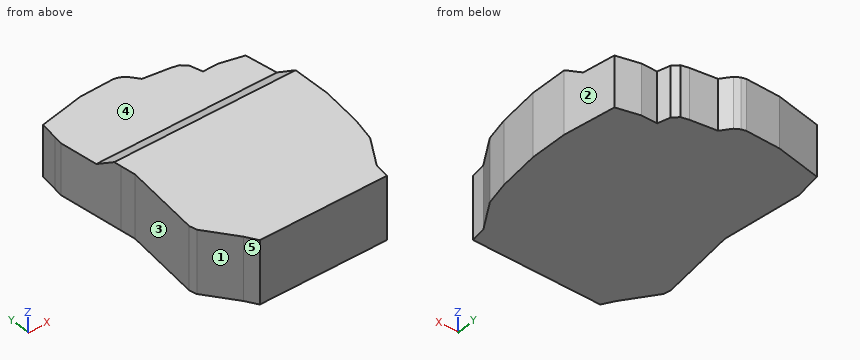
from build123d import *

# Parameters (mm, degrees)
BOSS_EXTRUDE1_DEPTH     = 30
CUT_EXTRUDE2_DEPTH      = 161.362841695
CUT_EXTRUDE2_DEPTH_BACK = 161.362841695


with BuildPart() as part:
    # Sketch1 → Boss-Extrude1 (new body)
    with BuildSketch(Plane.XY):
        Polygon((546.580924534, 9.896085679), (608.250924534, 9.896085679), (609.468725462, 17.325239217), (618.364062826, 31.698748766), (621.209508482, 43.308723045), (623.868380606, 63.224196603), (623.868380606, 81.054488799), (620.357339754, 106.059490311), (609.468725462, 108.728140515), (601.88762533, 108.728140515), (600.342350418, 114.668879106), (597.693307712, 117.244337292), (594.121848564, 118.119653006), (581.623216062, 119.788318601), (578.065152196, 124.442825109), (575.59297034, 125.972784898), (573.39799577, 126.510743097), (557.030037078, 126.118131563), (535.309704018, 121.76025213), (533.883150006, 113.057607434), (533.173455584, 108.728140515), (536.320171406, 77.786869686), (537.054893461, 70.562437811), (532.098682684, 33.439447285), (532.810591456, 29.891185826), (543.388975695, 15.373727724), align=None)
    extrude(amount=BOSS_EXTRUDE1_DEPTH)

    # Sketch2 → Cut-Extrude2 (cut, two sides: drawn at the far end of the back side and taken through both)
    with BuildSketch(Plane(origin=(530, 0, 0), x_dir=(0, 0, -1), z_dir=(1, 0, 0)).offset(-CUT_EXTRUDE2_DEPTH_BACK)):
        Polygon((-24.212, 126.510743097), (-24.212, 90.610743097), (-30, 81.373139386), (-30, 126.510743097), align=None)
    extrude(amount=CUT_EXTRUDE2_DEPTH + CUT_EXTRUDE2_DEPTH_BACK, mode=Mode.SUBTRACT)


solid = part.part
Design review of the part built by this model. Coordinates are the model's own, in mm. Face numbers are marked on the shaded views. A direction names the side the tool comes from. Coordinates: 2 decimals unless noted, no trailing zeros. Loops run counter-clockwise (first coordinate to the right, second up) from the corner with the lowest first, then second, coordinate; pieces in that order, holes last. Notation, with made-up numbers: (11.5, -24) -> (70.5, -24) arc R23 ccw to (70.5, -9) -> close; hole circle Ø9 at (9.5, 83). An arc over 180 degrees is marked (long way). Use a Markdown table: item, result. Add a question column.
Item 1: We need section A-A, the plane z = 9.75. Write out the cut boundary in (x, y).
Item 2: We need section C-C, the plane y = 85. Write out the cut boundary in (x, z).
Item 3: We need section B-B, the plane x = 606.5. Write out the cut boundary in (y, z).
Item 4: Machinability: for the marked faces 4 and 5, which of the approach directions +Z, -Z, +X, -X, +Y, -Y give a long, thin tool a straight path to every point of the face, cutting with its end or side? Answer none if there is none.
Item 5: We need section D-D, the plane x = 561.5. Write out the cut boundary in (y, z).
Item 6: Clearance check with flat-ended pins moving along their axes: P1, Ø5, axis at y = 30.5, z = 8, coming from the -X side; P2, Ø11, axis at x = 586, y = 107.5, coming from the +Z side; P3, Ø8.5, axis at x = 604.5, z = 8, coming from the +Y side. State where each tip first meets the part, or that it passes through.
Item 7: Wall thickness on L1, parallel to Y at x = 607, z = 9.75; L2, parallel to Z at x = 614.5, y = 101; L3, parallel to Y at x = 617, z = 26.75: over which ranges is each line inside the solid? List them lowest first. Write a range as from..to.
Item 8: The part is to be moulded in two halves that separate along Y. For the marked faces 1, 2 and 3, say which applies: +Y half, -Y half, draft (parallel to the pull), parting line (faces both ways), or undercut.
Numbers:
| question | item | result |
|---|---|---|
| 1 | outline | (532.1, 33.44) -> (532.81, 29.89) -> (543.39, 15.37) -> (546.58, 9.9) -> (608.25, 9.9) -> (609.47, 17.33) -> (618.36, 31.7) -> (621.21, 43.31) -> (623.87, 63.22) -> (623.87, 81.05) -> (620.36, 106.06) -> (609.47, 108.73) -> (601.89, 108.73) -> (600.34, 114.67) -> (597.69, 117.24) -> (594.12, 118.12) -> (581.62, 119.79) -> (578.07, 124.44) -> (575.59, 125.97) -> (573.4, 126.51) -> (557.03, 126.12) -> (535.31, 121.76) -> (533.17, 108.73) -> (537.05, 70.56) -> close |
| 2 | outline | (535.59, 0) -> (623.31, 0) -> (623.31, 27.73) -> (535.59, 27.73) -> close |
| 3 | outline | (9.9, 0) -> (108.73, 0) -> (108.73, 24.21) -> (90.61, 24.21) -> (81.37, 30) -> (9.9, 30) -> close |
| 4 | face 4 | +Z, +X, -X, +Y |
| 4 | face 5 | +Z, -Z, -X, -Y |
| 5 | outline | (9.9, 0) -> (126.23, 0) -> (126.23, 24.21) -> (90.61, 24.21) -> (81.37, 30) -> (9.9, 30) -> close |
| 6 | P1 | stops at x = 532.19 |
| 6 | P2 | stops at z = 24.21 |
| 6 | P3 | stops at y = 114.76 |
| 7 | L1 | y = 9.9..108.73 |
| 7 | L2 | z = 0..24.21 |
| 7 | L3 | y = 29.49..86.56 |
| 8 | face 1 | -Y half |
| 8 | face 2 | +Y half |
| 8 | face 3 | undercut |
